```python
from build123d import *

# Parameters (mm, degrees)
SKETCH1_R           = 17.5
SKETCH1_R_2         = 15.1
BOSS_EXTRUDE1_DEPTH = 10
BOSS_EXTRUDE2_DEPTH = 4
SKETCH3_R           = 2.5
CUT_EXTRUDE1_DEPTH  = 4
SKETCH4_W           = 5
SKETCH4_H           = 8
CUT_EXTRUDE2_DEPTH  = 10
CHAMFER1_SIZE       = 5


with BuildPart() as part:
    # Sketch1 → Boss-Extrude1 (new body)
    with BuildSketch(Plane.XY):
        Circle(SKETCH1_R)
        Circle(SKETCH1_R_2, mode=Mode.SUBTRACT)
    extrude(amount=BOSS_EXTRUDE1_DEPTH)

    # Sketch2 → Boss-Extrude2 (add)
    with BuildSketch(Plane(origin=(0, 0, 0), x_dir=(-1, 0, 0), z_dir=(0, 0, -1))):
        with BuildLine():
            Line((14.361406616, 10), (35, 10))
            Line((35, 10), (35, -10))
            Line((35, -10), (14.361406616, -10))
            ThreePointArc((14.361406616, -10), (0, -17.5), (-14.361406616, -10))
            Line((-14.361406616, -10), (-35, -10))
            Line((-35, -10), (-35, 10))
            Line((-35, 10), (-14.361406616, 10))
            ThreePointArc((-14.361406616, 10), (0, 17.5), (14.361406616, 10))
        make_face()
    extrude(amount=BOSS_EXTRUDE2_DEPTH)

    # Sketch3 → Cut-Extrude1 (cut)
    with BuildSketch(Plane.XY):
        with Locations((-27, 0)):
            Circle(SKETCH3_R)
        with Locations((27, 0)):
            Circle(SKETCH3_R)
    extrude(amount=-CUT_EXTRUDE1_DEPTH, mode=Mode.SUBTRACT)

    # Sketch4 → Cut-Extrude2 (cut)
    with BuildSketch(Plane.XY.offset(10)):
        with Locations((0, 15.1)):
            Rectangle(SKETCH4_W, SKETCH4_H)
    extrude(amount=-CUT_EXTRUDE2_DEPTH, mode=Mode.SUBTRACT)

    # Chamfer1
    chamfer1_edges = [part.edges().sort_by_distance(p)[0] for p in [
        (2.5, 16.106058225, 10),
        (-2.5, 16.106058225, 10),
    ]]
    chamfer(chamfer1_edges, length=CHAMFER1_SIZE)


solid = part.part
```
The model under review builds one solid part; all positions refer to its coordinate system, in mm. A direction names the side the tool comes from. Give positions to 0.01 mm unless a question says otherwise; leave off trailing zeros. Loops run counter-clockwise (first coordinate to the right, second up) from the corner with the lowest first, then second, coordinate; pieces in that order, holes last. Notation, with made-up numbers: (-13, 3) -> (9, 3) arc R17 cw to (9, 7) -> close; hole circle Ø11 at (55.5, 85.5). An arc over 180 degrees is marked (long way). Use CSV: the item, a comma, the result in double quotes.
1. Consider section B-B, the plane y = 0. Write out the cut boundary in (x, z).
Result:
outline,"(-35, -4) -> (-29.5, -4) -> (-29.5, 0) -> (-35, 0) -> close; (-24.5, -4) -> (24.5, -4) -> (24.5, 0) -> (17.5, 0) -> (17.5, 10) -> (15.1, 10) -> (15.1, 0) -> (-15.1, 0) -> (-15.1, 10) -> (-17.5, 10) -> (-17.5, 0) -> (-24.5, 0) -> close; (29.5, -4) -> (35, -4) -> (35, 0) -> (29.5, 0) -> close"
2. Machinability: for faces 5 (the face through (-25, -10, -2)), 6 (the face through (-25, 10, -2)), 7 (the face through (2.5, 16, 3)), 8 (the face through (-0.629, -15.087, 4.93)), which of the approach directions +Z, -Z, +X, -X, +Y, -Y give a long, thin tool a straight path to every point of the face, cutting with its end or side? Answer none if there is none.
Result:
face 5,"+Z, -Z, -X, -Y"
face 6,"+Z, -Z, -X, +Y"
face 7,"+Z, +Y"
face 8,"+Z"
3. Consider section A-A, the plane x = 27. Write out the cut boundary in (y, z).
Result:
outline,"(-10, -4) -> (-2.5, -4) -> (-2.5, 0) -> (-10, 0) -> close; (2.5, -4) -> (10, -4) -> (10, 0) -> (2.5, 0) -> close"
4. Consider section D-D, the plane y = -4. Write out the cut boundary in (x, z), then the cut area to 3 significant figures.
Result:
outline,"(-35, -4) -> (35, -4) -> (35, 0) -> (17.04, 0) -> (17.04, 10) -> (14.56, 10) -> (14.56, 0) -> (-14.56, 0) -> (-14.56, 10) -> (-17.04, 10) -> (-17.04, 0) -> (-35, 0) -> close"
area,"330 mm²"
5. To check wall thickness, follow probe 1 along X at (y, z) = (0, 2.25); probe 2 along Z at (x, y) = (-21.5, 2.5); probe 3 along Y at (x, z) = (31.5, -0.25). State the ranges of each line that lie inside material, in increasing order. Write a range as from..to.
Result:
probe 1,"x = -17.5..-15.1, 15.1..17.5"
probe 2,"z = -4..0"
probe 3,"y = -10..10"
6. Consider section C-C, the plane z = -2.25. Write out the cut boundary in (x, y).
Result:
outline,"(-35, -10) -> (-14.36, -10) arc R17.5 ccw to (14.36, -10) -> (35, -10) -> (35, 10) -> (14.36, 10) arc R17.5 ccw to (-14.36, 10) -> (-35, 10) -> close; hole circle Ø5 at (-27, 0); hole circle Ø5 at (27, 0)"
7. For P1, Ø2, axis at x = 19, z = 0, coming from the -Y side; P2, Ø1.5, axis at y = -9, z = 3.5, coming from the +X side; P3, Ø1.2, axis at x = -21, z = -2.5, coming from the +Y side; P4, Ø6.5, axis at x = -27, y = 0, coming from the -Z side, all flat-tipped, find the tip position at first contact; note any pin that passes through.
Result:
P1,"stops at y = -10"
P2,"stops at x = 15.43"
P3,"stops at y = 10"
P4,"stops at z = -4"
8. The part is to be moulded in two halves that separate along Y. For faces 1 (the face through (25, 10, -2)), 2 (the face through (0, 1, 0)), 3 (the face through (25, -10, -2)), 4 (the face through (-2.5, 16, 3)), say which applies: +Y half, -Y half, draft (parallel to the pull), parting line (faces both ways), or undercut.
Result:
face 1,"+Y half"
face 2,"undercut"
face 3,"-Y half"
face 4,"draft"
